Design review of the part built by this model. Coordinates are the model's own, in mm. Face numbers are marked on the shaded views. A direction names the side the tool comes from. Coordinates: 2 decimals unless noted, no trailing zeros. Loops run counter-clockwise (first coordinate to the right, second up) from the corner with the lowest first, then second, coordinate; pieces in that order, holes last. Notation, with made-up numbers: (3.5, 69) -> (17.5, 69) arc R19 ccw to (17.5, 87) -> close; hole circle Ø10 at (22.5, 25). An arc over 180 degrees is marked (long way). Use one line per item in the form item = value. Start each with the question number.
1. Consider section B-B (z = -3.75). State the section outline as (x, y) points (3 decimals), then the cut area to 3 significant figures.
2. Consider section C-C (x = -1.5). State the section outline as (y, z) points.
3. Consider section A-A (y = -1.5). State the section outline as (x, z) points.
4. The part is to be moulded in two halves that separate along X. For the marked faces 1, 2, 3 and 4, say which applies: released by +X, released by -X, zero draft, split by the parting line, or undercut.
5. For pin 1 (4 mm diameter, centred on x = 2, y = -8, fed in from -Z); pin 2 (0.7 mm diameter, centred on y = 2.5, z = -9, fed in from -X) (3 decimals); pin 3 (8 mm diameter, centred on x = -1, z = 1, fed in from -Y); pin 4 (0.5 mm diameter, centred on y = -13, z = 9, fed in from +X) (3 decimals), all flat-tipped, find the tip position at first contact; note any pin that passes through.
6. Machinability: for the marked faces 5, 6, 7 and 8, which of the approach directions +Z, -Z, +X, -X, +Y, -Y give a long, thin tool a straight path to every point of the face, cutting with its end or side? Answer none if there is none.
7. Wall thickness on line 1 (X direction, y = -7.5, z = 0); line 2 (Y direction, x = -4.75, z = -4.25); line 3 (Z direction, x = -6.25, y = -0.25): over which ranges is each line inside the solid? List them lowest first. Write a range as from..to.
8. Consider section D-D (z = 0.25). State the section outline as (x, y) points, then the cut area to 3 significant figures.
from build123d import *

# Parameters (mm, degrees)
ESQUISSE1_W             = 15.3
ESQUISSE1_H             = 20.4
BOSS_EXTRU_1_DEPTH      = 1.6
ESQUISSE2_W             = 2.5
ESQUISSE2_H             = 20.32
BOSS_EXTRU_2_DEPTH      = 10.9
BOSS_EXTRU_3_DEPTH      = 3
BOSS_EXTRU_3_DEPTH_BACK = 13.9
ESQUISSE3_W             = 0.65
ESQUISSE3_H             = 0.65
ESQUISSE4_W             = 5
ESQUISSE4_H             = 5
ESQUISSE4_W_2           = 3
ESQUISSE4_H_2           = 3
BOSS_EXTRU_4_DEPTH      = 1


with BuildPart() as part:
    # Esquisse1 → Boss.-Extru.1 (new body)
    with BuildSketch(Plane(origin=(0, 0, 0), x_dir=(1, 0, 0), z_dir=(0, 1, 0))):
        Rectangle(ESQUISSE1_W, ESQUISSE1_H)
    extrude(amount=BOSS_EXTRU_1_DEPTH)

    # Esquisse2 → Boss.-Extru.2 (add)
    with BuildSketch(Plane(origin=(0, 0, 0), x_dir=(1, 0, 0), z_dir=(0, 1, 0))):
        with Locations((-6.35, 0)):
            Rectangle(ESQUISSE2_W, ESQUISSE2_H)
        with Locations((6.35, 0)):
            Rectangle(ESQUISSE2_W, ESQUISSE2_H)
    extrude(amount=-BOSS_EXTRU_2_DEPTH)

    # Esquisse3 → Boss.-Extru.3 (add, two sides: drawn at the far end of the back side and taken through both)
    with BuildSketch(Plane.XZ.offset(10.9).offset(-BOSS_EXTRU_3_DEPTH_BACK)):
        with Locations((-6.35, 1.27)):
            Rectangle(ESQUISSE3_W, ESQUISSE3_H)
        with Locations((-6.35, -1.27)):
            Rectangle(ESQUISSE3_W, ESQUISSE3_H)
        with Locations((-6.35, 3.81)):
            Rectangle(ESQUISSE3_W, ESQUISSE3_H)
        with Locations((-6.35, 6.35)):
            Rectangle(ESQUISSE3_W, ESQUISSE3_H)
        with Locations((-6.35, 8.89)):
            Rectangle(ESQUISSE3_W, ESQUISSE3_H)
        with Locations((-6.35, -8.89)):
            Rectangle(ESQUISSE3_W, ESQUISSE3_H)
        with Locations((-6.35, -6.35)):
            Rectangle(ESQUISSE3_W, ESQUISSE3_H)
        with Locations((-6.35, -3.81)):
            Rectangle(ESQUISSE3_W, ESQUISSE3_H)
        with Locations((6.35, -8.89)):
            Rectangle(ESQUISSE3_W, ESQUISSE3_H)
        with Locations((6.35, -6.35)):
            Rectangle(ESQUISSE3_W, ESQUISSE3_H)
        with Locations((6.35, -3.81)):
            Rectangle(ESQUISSE3_W, ESQUISSE3_H)
        with Locations((6.35, 1.27)):
            Rectangle(ESQUISSE3_W, ESQUISSE3_H)
        with Locations((6.35, -1.27)):
            Rectangle(ESQUISSE3_W, ESQUISSE3_H)
        with Locations((6.35, 3.81)):
            Rectangle(ESQUISSE3_W, ESQUISSE3_H)
        with Locations((6.35, 6.35)):
            Rectangle(ESQUISSE3_W, ESQUISSE3_H)
        with Locations((6.35, 8.89)):
            Rectangle(ESQUISSE3_W, ESQUISSE3_H)
    extrude(amount=BOSS_EXTRU_3_DEPTH + BOSS_EXTRU_3_DEPTH_BACK)

    # Esquisse4 → Boss.-Extru.4 (add)
    with BuildSketch(Plane(origin=(0, 1.6, 0), x_dir=(1, 0, 0), z_dir=(0, 1, 0))):
        with Locations((0.061900131, 0.824485309)):
            Rectangle(ESQUISSE4_W, ESQUISSE4_H)
        with Locations((-2.4, -7.7)):
            Rectangle(ESQUISSE4_W_2, ESQUISSE4_H_2)
    extrude(amount=BOSS_EXTRU_4_DEPTH)


solid = part.part
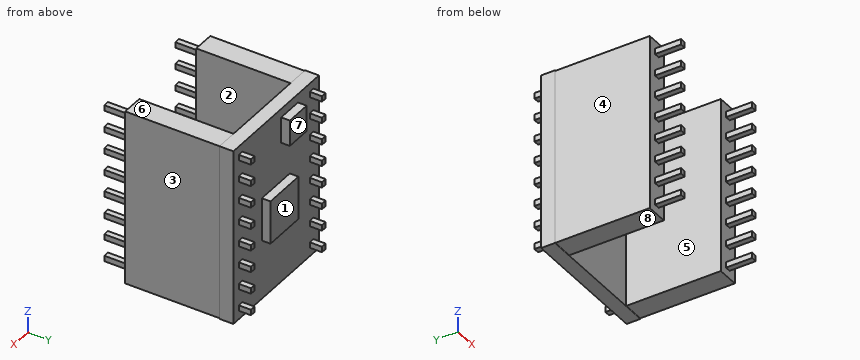
Geometry check:
q1.outline = (-7.65, 0) -> (-7.6, 0) -> (-7.6, -10.9) -> (-6.675, -10.9) -> (-6.675, -13.9) -> (-6.025, -13.9) -> (-6.025, -10.9) -> (-5.1, -10.9) -> (-5.1, 0) -> (5.1, 0) -> (5.1, -10.9) -> (6.025, -10.9) -> (6.025, -13.9) -> (6.675, -13.9) -> (6.675, -10.9) -> (7.6, -10.9) -> (7.6, 0) -> (7.65, 0) -> (7.65, 1.6) -> (6.675, 1.6) -> (6.675, 3) -> (6.025, 3) -> (6.025, 1.6) -> (-6.025, 1.6) -> (-6.025, 3) -> (-6.675, 3) -> (-6.675, 1.6) -> (-7.65, 1.6) -> close
q1.area = 84.7 mm²
q2.outline = (0, -10.2) -> (1.6, -10.2) -> (1.6, -3.32) -> (2.6, -3.32) -> (2.6, 1.68) -> (1.6, 1.68) -> (1.6, 6.2) -> (2.6, 6.2) -> (2.6, 9.2) -> (1.6, 9.2) -> (1.6, 10.2) -> (0, 10.2) -> close
q3.outline = (-7.6, -10.16) -> (-5.1, -10.16) -> (-5.1, 10.16) -> (-7.6, 10.16) -> close; (5.1, -10.16) -> (7.6, -10.16) -> (7.6, 10.16) -> (5.1, 10.16) -> close
q4.face_1 = undercut
q4.face_2 = undercut
q4.face_3 = released by +X
q4.face_4 = released by -X
q5.pin_1 = through
q5.pin_2 = -6.675
q5.pin_3 = 0
q5.pin_4 = 6.675
q6.face_5 = +Z, -Z, -Y
q6.face_6 = +Z, +X, -X, -Y
q6.face_7 = +Z, -Z, +Y
q6.face_8 = -Z, +X, -X, -Y
q7.line_1 = -7.6..-5.1, 5.1..7.6
q7.line_2 = 0..1.6
q7.line_3 = -10.16..10.16
q8.outline = (-7.65, 0) -> (-7.6, 0) -> (-7.6, -10.9) -> (-5.1, -10.9) -> (-5.1, 0) -> (5.1, 0) -> (5.1, -10.9) -> (7.6, -10.9) -> (7.6, 0) -> (7.65, 0) -> (7.65, 1.6) -> (2.56, 1.6) -> (2.56, 2.6) -> (-2.44, 2.6) -> (-2.44, 1.6) -> (-7.65, 1.6) -> close
q8.area = 84.0 mm²
